Design review of the part built by this model. Coordinates are the model's own, in mm. A direction names the side the tool comes from. Round coordinates to 2 decimals unless told otherwise and drop trailing zeros. Write each loop counter-clockwise with the first axis right and the second up, starting at its lowest first coordinate (ties: lowest second). Pieces come first, ordered by that corner, then holes. Notation, with made-up numbers: (89, 24.25) -> (114, 24.25) arc R16 cw to (114, 41.25) -> close; hole circle Ø3 at (57.5, -12). An arc over 180 degrees is marked (long way). Write item = value, one per line. Start each with the question number.
Item 1: Add section A-A, the plane z = 0.75. State the section outline as (x, y) points, then the cut area to 3 significant figures.
Item 2: Machinability: for faces 4 (the flat face through (49, 0, 0)), 5 (the flat face through (48.82, 60.62, 0.06)), which of the approach directions +Z, -Z, +X, -X, +Y, -Y give a long, thin tool a straight path to every point of the face, cutting with its end or side? Answer none if there is none.
Item 3: For pin 1 Ø1.5 at (x, z) = (63, 2) entering from +Y; pin 2 Ø1 at (x, z) = (60.5, 1) entering from +Y; pin 3 Ø2 at (y, z) = (59.5, 2.5) entering from +X; pin 4 Ø6 at (x, y) = (69.5, 66) entering from +Z, all flat-tipped, find the tip position at first contact; note any pin that passes through.
Item 4: Add section C-C, the plane y = 76. State the section outline as (x, z) points, then the cut area to 3 significant figures.
Item 5: Mouldability with a two-part tool opening along X and no side actions: class faces 1 (the flat face through (47, 16, 0)), 2 (the flat face through (49, 61, 4)), 3 (the flat face through (100, 5, 0)) as released by +X, released by -X, zero draft, split by the parting line, or undercut.
Item 6: To check wall thickness, follow L1, parallel to Y at x = 51.5, z = 3; L2, parallel to X at y = 88.5, z = -2; L3, parallel to Y at x = 41.5, z = 3.75. State the ranges of each line that lie inside material, in increasing order.
Item 7: Add section D-D, the plane x = 86. State the section outline as (y, z) points, then the cut area to 3 significant figures.
Item 8: Add section B-B, the plane x = 25. State the section outline as (y, z) points, then the cut area to 3 significant figures.
from build123d import *

# Parameters (mm, degrees)
EXTRUDE_1_DEPTH = 4


with BuildPart() as part:
    # 草图1 → 凸台-拉伸1 (new, symmetric)
    with BuildSketch(Plane.XY):
        Polygon((0, 0), (100, 0), (100, 10), (30, 120), (0, 120), align=None)
        Polygon((16, 104), (21.21686573, 104), (77.21686573, 16), (16, 16), align=None, mode=Mode.SUBTRACT)
    extrude(amount=EXTRUDE_1_DEPTH, both=True)


solid = part.part
Result set:
q1.outline = (0, 0) -> (100, 0) -> (100, 10) -> (30, 120) -> (0, 120) -> close; hole (16, 16) -> (77.22, 16) -> (21.22, 104) -> (16, 104) -> close
q1.area = 5,230 mm²
q2.face_4 = +Z, -Z, +X, -X, -Y
q2.face_5 = +Z, -Z
q3.pin_1 = 69.32
q3.pin_2 = 72.86
q3.pin_3 = 69.14
q3.pin_4 = through
q4.outline = (0, -4) -> (16, -4) -> (16, 4) -> (0, 4) -> close; (39.04, -4) -> (58, -4) -> (58, 4) -> (39.04, 4) -> close
q4.area = 280 mm²
q5.face_1 = undercut
q5.face_2 = zero draft
q5.face_3 = released by +X
q6.L1 = 0 to 16, 56.41 to 86.21
q6.L2 = 0 to 16, 31.08 to 50.05
q6.L3 = 0 to 16, 72.13 to 101.93
q7.outline = (0, -4) -> (32, -4) -> (32, 4) -> (0, 4) -> close
q7.area = 256 mm²
q8.outline = (0, -4) -> (16, -4) -> (16, 4) -> (0, 4) -> close; (98.06, -4) -> (120, -4) -> (120, 4) -> (98.06, 4) -> close
q8.area = 304 mm²
